For this review, take the finished solid that the model builds, in its own axes (mm). Face numbers are marked on the shaded views. Coordinates: 2 decimals unless noted, no trailing zeros. Write each loop counter-clockwise with the first axis right and the second up, starting at its lowest first coordinate (ties: lowest second). Pieces come first, ordered by that corner, then holes.
```python
from build123d import *

# Parameters (mm, degrees)
F1_DEPTH = 15
F3_D     = 5


with BuildPart() as f1:
    # F0 (on Top) → F1 (new body)
    with BuildSketch(Plane.XY):
        with BuildLine():
            Line((40, 0), (0, 0))
            Line((0, 0), (0, -19))
            Line((0, -19), (14.08392, -19))
            ThreePointArc((14.08392, -19), (20, -14), (25.91608, -19))
            Line((25.91608, -19), (40, -19))
            Line((40, -19), (40, 0))
        make_face()
    extrude(amount=F1_DEPTH)

    # F3 (through all)
    with Locations(Plane(origin=(0, 0, 0), x_dir=(-1, 0, 0), z_dir=(0, 1, 0))):
        with Locations((-8, 6.5), (-32, 6.5)):
            Hole(F3_D / 2)


solid = f1.part
```
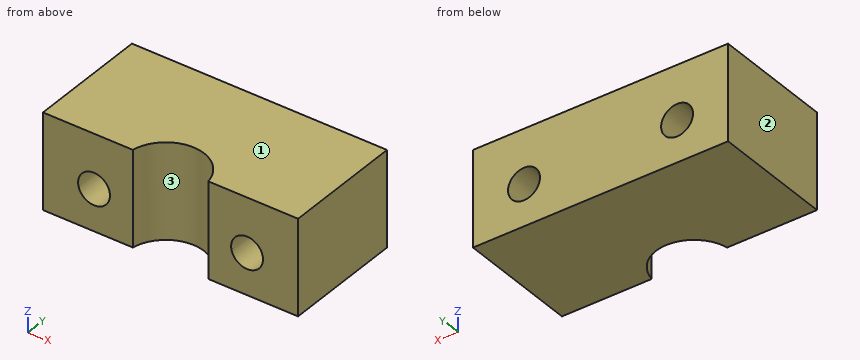
Q1. Draft analysis for pull direction X (two halves, no side actions). For the marked faces 1, 2 and 3, state which applies: +X half, -X half, draft (parallel to the pull), parting line (faces both ways), or undercut.
Ans:
face 1: draft
face 2: -X half
face 3: undercut
Q2. For probe 1 along Z at (x, y) = (8, -13); probe 2 along X at (y, z) = (-1.75, 5.25); probe 3 along Z at (x, y) = (8.5, -12.5), list the stretches that pass through material, from the lowest coordinate up.
Ans:
probe 1: z = 0 to 4, 9 to 15
probe 2: x = 0 to 5.83, 10.17 to 29.83, 34.17 to 40
probe 3: z = 0 to 4.05, 8.95 to 15
Q3. Add section D-D (x = 6.5). State the section outline as (y, z) points, then the cut area to 3 significant figures.
Ans:
outline: (-19, 0) - (0, 0) - (0, 4.5) - (-19, 4.5) - close; (-19, 8.5) - (0, 8.5) - (0, 15) - (-19, 15) - close
area: 209 mm2
Q4. Clearance check with flat-ended pins moving along their axes: pin 1 Ø1.5 at (x, z) = (20.5, 5.5) entering from -Y; pin 2 Ø4 at (y, z) = (-9, 9.5) entering from -X; pin 3 Ø4 at (x, z) = (8, 6.5) entering from +Y; pin 4 Ø5 at (x, z) = (22, 8) entering from -Y. State where each tip first meets the part, or that it passes through.
Ans:
pin 1: stops at y = -14.13
pin 2: stops at x = 0
pin 3: passes through
pin 4: stops at y = -16.03
Q5. Add section C-C (y = -16.25). State the section outline as (x, z) points.
Ans:
outline: (0, 0) - (15.32, 0) - (15.32, 15) - (0, 15) - close; (24.68, 0) - (40, 0) - (40, 15) - (24.68, 15) - close; hole circle Ø5 at (8, 6.5); hole circle Ø5 at (32, 6.5)
Q6. Add section A-A (x = 32). State the section outline as (y, z) points.
Ans:
outline: (-19, 0) - (0, 0) - (0, 4) - (-19, 4) - close; (-19, 9) - (0, 9) - (0, 15) - (-19, 15) - close
Q7. Add section B-B (z = 6.5). State the section outline as (x, y) points.
Ans:
outline: (0, -19) - (5.5, -19) - (5.5, 0) - (0, 0) - close; (10.5, -19) - (14.08, -19) arc R6 cw to (25.92, -19) - (29.5, -19) - (29.5, 0) - (10.5, 0) - close; (34.5, -19) - (40, -19) - (40, 0) - (34.5, 0) - close
